from build123d import *

# Parameters (mm, degrees)
SKETCH_R           = 20
SKETCH_R_2         = 3.05
PAD_DEPTH          = 1.7
SKETCH001_W        = 1.5
SKETCH001_H        = 8
POCKET_DEPTH       = 114.889162
POLARPATTERN_COUNT = 20
SKETCH002_R        = 12.023415
SKETCH002_R_2      = 3.05
PAD001_DEPTH       = 1.3


with BuildPart() as part:
    # Sketch → Pad (new body)
    with BuildSketch(Plane.XY):
        Circle(SKETCH_R)
        Circle(SKETCH_R_2, mode=Mode.SUBTRACT)
    extrude(amount=PAD_DEPTH)

    # Sketch001 (on Face4 of Pad) → Pocket (cut, through all)
    with BuildSketch(Plane.XY.offset(1.7)):
        with Locations((0, 16)):
            Rectangle(SKETCH001_W, SKETCH001_H)
    pocket = extrude(amount=-POCKET_DEPTH, mode=Mode.SUBTRACT)

    # PolarPattern: Pocket ×20 about axis
    polarpattern_axis = Axis((0, 0, 1.7), (0, 0, 1))
    for i in range(1, POLARPATTERN_COUNT):
        add(pocket.rotate(polarpattern_axis, i * 360 / POLARPATTERN_COUNT), mode=Mode.SUBTRACT)

    # Sketch002 (on Face4 of PolarPattern) → Pad001 (join)
    with BuildSketch(Plane.XY.offset(1.7)):
        Circle(SKETCH002_R)
        Circle(SKETCH002_R_2, mode=Mode.SUBTRACT)
    extrude(amount=PAD001_DEPTH)


solid = part.part
Can you work these out from the model? Positions are in its coordinate system, mm. A direction names the side the tool comes from. Coordinates: 2 decimals unless noted, no trailing zeros. Loops run counter-clockwise (first coordinate to the right, second up) from the corner with the lowest first, then second, coordinate; pieces in that order, holes last. Notation, with made-up numbers: M 21.5,-21.5 L 27.5,-21.5 A29 cw 27.5,4.5 Z; hole C 11,-39 d5. An arc over 180 degrees is marked long. Answer as CSV lines item,"result". Start each with the question number.
1. For pin 1 Ø3.5 at (x, y) = (6.5, -16) entering from +Z; pin 2 Ø1 at (x, z) = (13.5, 0.5) entering from +Y; pin 3 Ø0.8 at (y, z) = (0, 0.5) entering from +X; pin 4 Ø1.5 at (x, y) = (-12.5, 15) entering from -Z, each with a flat end and sliding along its axis, tell me the tip position at first contact or that it passes through.
2. Suppose I cut it at D-D, the plane x = 5. List the corners of the cut face in (y, z) for me, plus the area to 3 significant figures.
3. Thinking about a two-plate mould opening in X: for faces 4 (the face through (-12, 0, 1)), 5 (the face through (-12, 12, 1.7)), 6 (the face through (11.47, 3.61, 2.34)), 7 (the face through (-3.047, 0.134, 1.479)), which applies, +X half, -X half, draft (parallel to the pull), parting line (faces both ways), or undercut?
4. For faces 1 (the face through (-5.64, 14.93, 0.86)), 2 (the face through (9.11, 17.805, 0.838)), 3 (the face through (12, 12, 1.7)), which set-ups out of +Z, -Z, +X, -X, +Y, -Y let a thin tool reach every point of the face, with its end or its side?
5. Suppose I cut it at C-C, the plane y = 14.5. List the corners of the cut face in (x, z) for me.
6. If I drill on probe 1 along Y at (x, z) = (0, 1.55); probe 2 along X at (y, z) = (9, 1.2); probe 3 along Y at (x, z) = (-13.5, 0.25), over which ranges is the centre line in solid material (lowest first)? Write a range as [from, to].
Output:
1,pin 1,"stops at z = 1.7"
1,pin 2,"stops at y = 15.2"
1,pin 3,"stops at x = 12"
1,pin 4,"stops at z = 0"
2,outline,"M -19.36,0 L -17.82,0 L -17.82,1.7 L -19.36,1.7 Z; M -12.96,0 L 12.96,0 L 12.96,1.7 L 10.93,1.7 L 10.93,3 L -10.93,3 L -10.93,1.7 L -12.96,1.7 Z; M 17.82,0 L 19.36,0 L 19.36,1.7 L 17.82,1.7 Z"
2,area,"77.8 mm^2"
3,face 4,"-X half"
3,face 5,"draft"
3,face 6,"parting line"
3,face 7,"undercut"
4,face 1,"+Z, -Z"
4,face 2,"+Z, -Z, +X, +Y"
4,face 3,"+Z, +X, +Y"
5,outline,"M -13.77,0 L -11.46,0 L -11.46,1.7 L -13.77,1.7 Z; M -9.61,0 L -5.5,0 L -5.5,1.7 L -9.61,1.7 Z; M -3.92,0 L -0.75,0 L -0.75,1.7 L -3.92,1.7 Z; M 0.75,0 L 3.92,0 L 3.92,1.7 L 0.75,1.7 Z; M 5.5,0 L 9.61,0 L 9.61,1.7 L 5.5,1.7 Z; M 11.46,0 L 13.77,0 L 13.77,1.7 L 11.46,1.7 Z"
6,probe 1,"y = [-12, -3.05], [3.05, 12]"
6,probe 2,"x = [-17.86, -13.66], [-11.11, 11.11], [13.66, 17.86]"
6,probe 3,"y = [-14.76, -10.74], [-8.88, -5.18], [-3.6, -0.75], [0.75, 3.6], [5.18, 8.88], [10.74, 14.76]"
